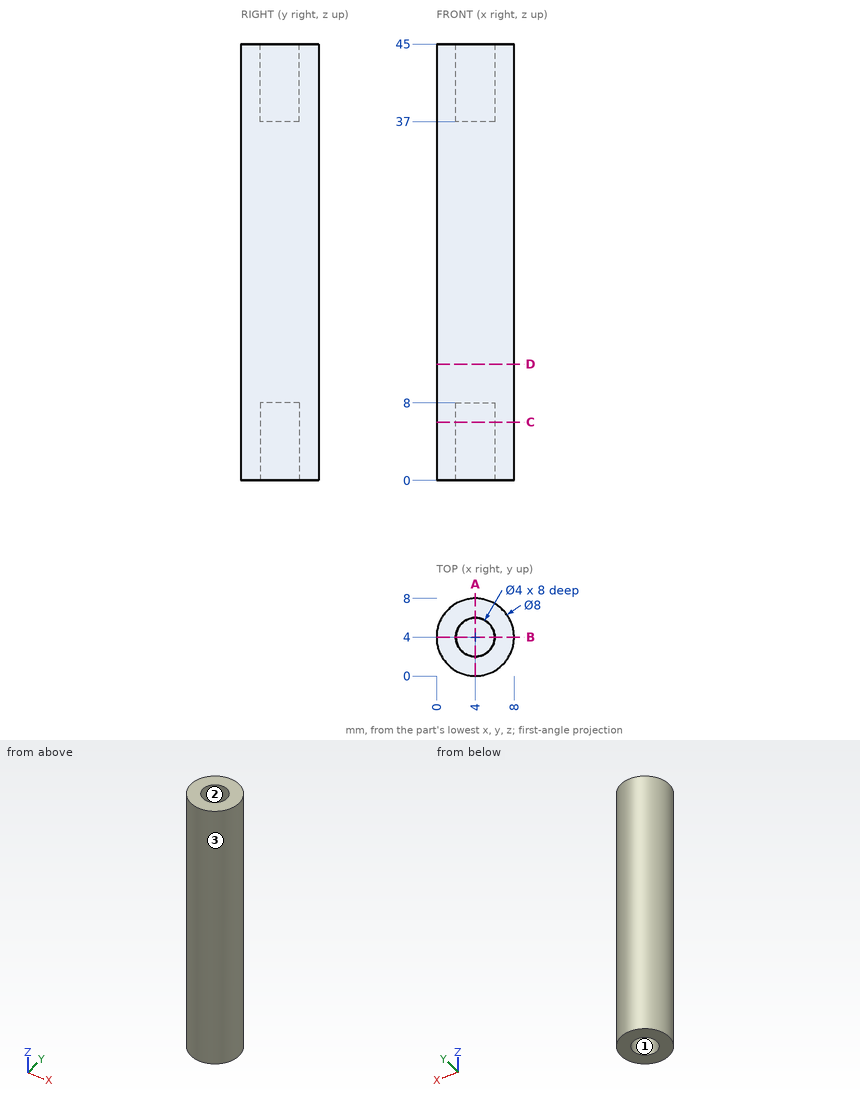
Verification items for this drawing (mm, ordinates from the low corner). Round coordinates to 2 decimals unless told otherwise and drop trailing zeros. Order: outer loops, then holes, each group sorted by start corner. A loop starts at its lowest first (then second) coordinate and runs counter-clockwise, first axis right, second up. Notation, with made-up numbers: M 22,48.25 L 68,48.25 A12 cw 68,68.25 Z; hole C 5.5,79 d8. An arc over 180 degrees is marked long. Answer in a Markdown table with one row per item. Add a question column.
Item 1: Depth check by flat-ended pin: pin 1 Ø1.5 at (x, z) = (2.5, 34.5) entering from +Y; pin 2 Ø1.2 at (x, y) = (4, 4.5) entering from +Z; pin 3 Ø1.5 at (y, z) = (1.5, 17) entering from +X. Enter the tip coordinate at first touch or a pass-through.
Item 2: Sectioned sample at A-A, the plane x = 4. Enter the section's corners in (y, z).
Item 3: Material ranges on L1, parallel to Y at x = 4, z = 3.75; L2, parallel to Z at x = 4.25, y = 2.5; L3, parallel to X at y = 3.75, z = 37.5, recorded low to high. Write a range as [from, to].
Item 4: Sectioned sample at D-D, the plane z = 12. Enter the section's corners in (x, y), plus the area to 3 significant figures.
Item 5: Draft check along Y on the marked faces 1, 2 and 3. Enter one of: released by +Y, released by -Y, zero draft, split by the parting line, or undercut.
Item 6: Sectioned sample at C-C, the plane z = 6. Enter the section's corners in (x, y), plus the area to 3 significant figures.
Filled in:
| question | item | result |
|---|---|---|
| 1 | pin 1 | stops at y = 7.93 |
| 1 | pin 2 | stops at z = 37 |
| 1 | pin 3 | stops at x = 7.6 |
| 2 | outline | M 0,0 L 2,0 L 2,8 L 6,8 L 6,0 L 8,0 L 8,45 L 6,45 L 6,37 L 2,37 L 2,45 L 0,45 Z |
| 3 | L1 | y = [0, 2], [6, 8] |
| 3 | L2 | z = [8, 37] |
| 3 | L3 | x = [0.01, 2.02], [5.98, 7.99] |
| 4 | outline | C 4,4 d8 |
| 4 | area | 50.3 mm² |
| 5 | face 1 | undercut |
| 5 | face 2 | undercut |
| 5 | face 3 | split by the parting line |
| 6 | outline | C 4,4 d8; hole C 4,4 d4 |
| 6 | area | 37.7 mm² |
